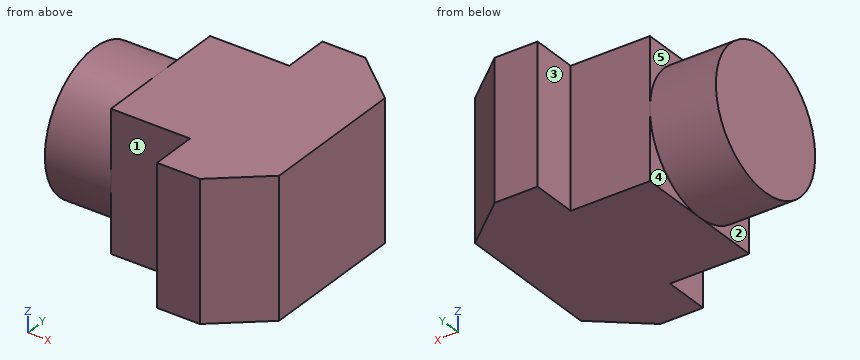
Autodesk Inventor part; units mm, degrees
ref_plane "YZ Plane" through (0, 0, 0) normal (1, 0, 0) x (0, 1, 0)
ref_plane "XZ Plane" through (0, 0, 0) normal (0, 1, 0) x (-1, 0, 0)
ref_plane "XY Plane" through (0, 0, 0) normal (0, 0, 1) x (1, 0, 0)
sketch "Sketch1" plane through (0, 0, 0) normal (0, 0, 1) x (1, 0, 0)
  line L0 (0, 10.5) -> (12, 10.5)
  line L1 (12, 10.5) -> (12, 17.5)
  line L2 (12, 17.5) -> (18.5, 17.5)
  line L3 (18.5, 17.5) -> (26, 11.2068)
  line L4 (0, 10.5) -> (0, -10.5)
  line L5 (0, -10.5) -> (12, -10.5)
  line L6 (12, -10.5) -> (12, -17.5)
  line L7 (12, -17.5) -> (18.5, -17.5)
  line L8 (18.5, -17.5) -> (26, -11.2068)
  line L9 (26, -11.2068) -> (26, 11.2068)
  point P0 (0, 0)
  point P1 (0, 0)
  dimension "d0" = 12
  dimension "d1" = 7
  dimension "d2" = 6.5
  dimension "d3" = 21
  dimension "d5" = 14
  dimension "d8" = 140
  dimension "d9" = 140
extrude "Extrusion1" add sketch "Sketch1" along normal blind 21
sketch "Sketch2" plane through (0, -10.5, 0) normal (-1, 0, 0) x (0, 0, 1)
  line L0 (0, 21) -> (0, 0)
  line L1 (0, 21) -> (0, 0)
  line L2 (0, 0) -> (21, 0)
  line L3 (21, 21) -> (21, 0)
  line L4 (0, 21) -> (21, 21)
  circle A0 centre (10.5, 10.5) radius 10.5
  point P0 (0, 10.5)
extrude "Extrusion2" add sketch "Sketch2" along normal blind 10 contours A0
equation "\"d9\" = d8"
properties part number "m_Schienenteil"
CAD build for the part. Positions are in the model's coordinates, mm. Face numbers are marked on the shaded views. A direction names the side the tool comes from. Round coordinates to 2 decimals unless told otherwise and drop trailing zeros. Order: outer loops, then holes, each group sorted by start corner. A loop starts at its lowest first (then second) coordinate and runs counter-clockwise, first axis right, second up. Notation, with made-up numbers: (51.5, 3) - (91.5, 3) arc R36 ccw to (91.5, 38) - close; hole circle Ø9 at (64.25, -3.75). An arc over 180 degrees is marked (long way). Answer as CSV lines item,"result". Start each with the question number.
1. Saw through at B-B, the plane y = -8. Write the cut outline in (x, z).
2. Saw through at A-A, the plane z = 9.5. Write the cut outline in (x, y).
3. Saw through at C-C, the plane x = 20.5. Write the cut outline in (y, z), and give its area (3 significant figures).
4. Drill centre lines: L1, parallel to Y at x = 0.5, z = 19.25; L2, parallel to Y at x = 23, z = 10.25; L3, parallel to X at y = -9.5, z = 18.5. Where is each one in solid material? Low to high. Write a range as [from, to].
5. Tool access for the marked faces 1, 2, 3, 4 and 5: list every direction of +Z, -Z, +X, -X, +Y, -Y with a clear straight run to the whole face (end or side of a thin tool).
6. Pin check, flat tips, straight feed: pin 1 (3.5 mm diameter, centred on y = -14, z = 6, fed in from -X); pin 2 (4 mm diameter, centred on x = -2, y = -2, fed in from -Z); pin 3 (12 mm diameter, centred on x = -5, z = 6.5, fed in from +Y); pin 4 (2 mm diameter, centred on x = -2.5, y = 10, fed in from +Z). Stop position of each tip, or through.
7. Saw through at D-D, the plane z = 18.5. Write the cut outline in (x, y).
Model answer:
1,outline,"(-10, 3.7) - (0, 3.7) - (0, 0) - (26, 0) - (26, 21) - (0, 21) - (0, 17.3) - (-10, 17.3) - close"
2,outline,"(-10, -10.45) - (0, -10.45) - (0, -10.5) - (12, -10.5) - (12, -17.5) - (18.5, -17.5) - (26, -11.21) - (26, 11.21) - (18.5, 17.5) - (12, 17.5) - (12, 10.5) - (0, 10.5) - (0, 10.45) - (-10, 10.45) - close"
3,outline,"(-15.82, 0) - (15.82, 0) - (15.82, 21) - (-15.82, 21) - close"
3,area,"665 mm²"
4,L1,"y = [-10.5, 10.5]"
4,L2,"y = [-13.72, 13.72]"
4,L3,"x = [0, 26]"
5,face 1,"+Z, -Z, -X, -Y"
5,face 2,"-Z, -X, -Y"
5,face 3,"+Z, -Z, -X, +Y"
5,face 4,"-Z, -X, +Y"
5,face 5,"+Z, -X, +Y"
6,pin 1,"stops at x = 12"
6,pin 2,"stops at z = 0"
6,pin 3,"stops at y = 10.5"
6,pin 4,"stops at z = 15.91"
7,outline,"(-10, -6.8) - (0, -6.8) - (0, -10.5) - (12, -10.5) - (12, -17.5) - (18.5, -17.5) - (26, -11.21) - (26, 11.21) - (18.5, 17.5) - (12, 17.5) - (12, 10.5) - (0, 10.5) - (0, 6.8) - (-10, 6.8) - close"
